Check sheet for the modelled part. Datum: model origin and axes. Units: mm. Face numbers are marked on the shaded views. A direction names the side the tool comes from. Coordinates: 2 decimals unless noted, no trailing zeros. Write each loop counter-clockwise with the first axis right and the second up, starting at its lowest first coordinate (ties: lowest second). Pieces come first, ordered by that corner, then holes. Notation, with made-up numbers: M 35.5,23 L 60.5,23 A31 cw 60.5,62 Z; hole C 71.25,33 d7. An arc over 180 degrees is marked long. Answer as CSV lines item,"result". Start each with the question number.
Q1. Thickness scan on line 1 along Z through (x, y) = (0, 6) (3 decimals); line 2 along Z through (x, y) = (0, 8.25) (3 decimals); line 3 along Y through (x, z) = (-2, 0) (1 decimal). Record the ranges inside material, lowest first. Write a range as from..to.
Q2. Sectioned sample at A-A, the plane y = 22.5. Record the cut outline in (x, z) (3 decimals).
Q3. Sectioned sample at D-D, the plane y = 63. Record the cut outline in (x, z) (1 decimal), then the cut area to 3 significant figures.
Q4. Depth check by flat-ended pin: pin 1 Ø18 at (y, z) = (65, 0.5) entering from -X; pin 2 Ø18 at (y, z) = (64, 5) entering from +X; pin 3 Ø8 at (x, z) = (-3.5, -4) entering from -Y. Enter the tip coordinate at first touch or a pass-through.
Q5. Mould release check, pull along Z, two halves, no side actions. Record for the marked faces 3, 4, 5 and 6: pulls with the +Z half, pulls with the -Z half, needs draft (parallel to the pull), parting line crosses it, or undercut.
Q6. Sectioned sample at C-C, the plane x = 0. Record the cut outline in (y, z) (1 decimal), then the cut area to 3 significant figures.
Q7. Access from +Z, -Z, +X, -X, +Y, -Y to the whole of each face (thin tool, end or side, straight path). Record for the marked faces 1 and 2.
Autodesk Fusion 360 part; units mm, degrees
sketch "Sketch1" plane through (0, 0, 0) normal (0, 1, 0) x (1, 0, 0)
  circle A0 centre (0, 0) radius 24.875
  line L0 (-23.4897, 87.6649) -> (23.4897, 87.6649)
  line L1 (23.4897, 87.6649) -> (64.1752, 64.1752)
  line L2 (64.1752, 64.1752) -> (87.6649, 23.4897)
  line L3 (87.6649, 23.4897) -> (87.6649, -23.4897)
  line L4 (87.6649, -23.4897) -> (64.1752, -64.1752)
  line L5 (64.1752, -64.1752) -> (23.4897, -87.6649)
  line L6 (23.4897, -87.6649) -> (-23.4897, -87.6649)
  line L7 (-23.4897, -87.6649) -> (-64.1752, -64.1752)
  line L8 (-64.1752, -64.1752) -> (-87.6649, -23.4897)
  line L9 (-87.6649, -23.4897) -> (-87.6649, 23.4897)
  line L10 (-87.6649, 23.4897) -> (-64.1752, 64.1752)
  line L11 (-64.1752, 64.1752) -> (-23.4897, 87.6649)
  line L12 (-87.6649, 0) -> (0, 0) construction
  line L13 (0, 0) -> (87.6649, 0) construction
  line L14 (0, 0) -> (0, -87.6649) construction
  line L15 (0, 0) -> (0, 87.6649) construction
  line L16 (-22.15, 82.6649) -> (22.15, 82.6649)
  line L17 (22.15, 82.6649) -> (60.5149, 60.5149)
  line L18 (60.5149, 60.5149) -> (82.6649, 22.15)
  line L19 (82.6649, 22.15) -> (82.6649, -22.15)
  line L20 (82.6649, -22.15) -> (60.5149, -60.5149)
  line L21 (60.5149, -60.5149) -> (22.15, -82.6649)
  line L22 (22.15, -82.6649) -> (-22.15, -82.6649)
  line L23 (-22.15, -82.6649) -> (-60.5149, -60.5149)
  line L24 (-60.5149, -60.5149) -> (-82.6649, -22.15)
  line L25 (-82.6649, -22.15) -> (-82.6649, 22.15)
  line L26 (-82.6649, 22.15) -> (-60.5149, 60.5149)
  line L27 (-60.5149, 60.5149) -> (-22.15, 82.6649)
  line L28 (0, 0) -> (-82.6649, 0) construction
  line L29 (0, 0) -> (0, 82.6649) construction
  line L30 (0, 0) -> (82.6649, 0) construction
  line L31 (0, 0) -> (0, -82.6649) construction
  point P0 (24.875, 0)
  dimension "d1" = 49.75
  dimension "d3" = 150
  dimension "d4" = 62.7899
  dimension "d5" = 5
  dimension "d9" = 150
  dimension "d10" = 44.3
extrude "Extrude1" add sketch "Sketch1" along normal blind 8 contours L16 L17 L18 L19 L20 L21 L22 L23 L24 L25 L26 L27
extrude "Extrude6" add sketch "Sketch1" along normal blind 28 contours L0 L1 L2 L3 L4 L5 L6 L7 L8 L9 L10 L11
extrude "Extrude2" add sketch "Sketch1" along normal blind 33 contours A0
sketch "Sketch2" plane through (0, 33, 0) normal (0, 1, 0) x (-1, 0, 0)
  circle A0 centre (0, 0) radius 24.875
  circle A1 centre (0, 0) radius 12.4375
  dimension "d15" = 49.75
  dimension "d16" = 24.875
extrude "Extrude3" add sketch "Sketch2" along normal blind 20 contours A1
sketch "Sketch3" plane through (0, 0, 0) normal (1, 0, 0) x (0, 0, -1)
  line L0 (12.4375, 53) -> (-12.4375, 53)
  line L1 (-12.4375, 33) -> (12.4375, 33)
  line L2 (0, 53) -> (0, 65.4375) construction
  circle A0 centre (0, 65.4375) radius 12.4375
  circle A1 centre (0, 65.4375) radius 8
  line L3 (0, 65.4375) -> (-12.4375, 65.4375) construction
  line L4 (0, 65.4375) -> (12.4375, 65.4375) construction
  line L5 (-12.4375, 65.4375) -> (-12.4375, 53)
  line L6 (12.4375, 65.4375) -> (12.4375, 53)
  dimension "d19" = 24.875
  dimension "d20" = 16
  dimension "d21" = 24.875
extrude "Extrude4" add sketch "Sketch3" along normal mid plane 10
extrude "Extrude5" cut 1 faces at (20.5903, 33, 1.8537) along direction (0, 1, 0) blind 50
fillet "Fillet1" radius 2 2 edges at (5, 53, 0) (-5, 53, 0)
sketch "Sketch4" plane through (0, 0, 0) normal (0, -1, 0) x (1, 0, 0)
  line L0 (-87.6649, -23.4897) -> (-64.1752, -64.1752)
  line L1 (-64.1752, -64.1752) -> (-23.4897, -87.6649)
  line L2 (-23.4897, -87.6649) -> (23.4897, -87.6649)
  line L3 (23.4897, -87.6649) -> (64.1752, -64.1752)
  line L4 (64.1752, -64.1752) -> (87.6649, -23.4897)
  line L5 (87.6649, -23.4897) -> (87.6649, 23.4897)
  line L6 (87.6649, 23.4897) -> (64.1752, 64.1752)
  line L7 (64.1752, 64.1752) -> (23.4897, 87.6649)
  line L8 (23.4897, 87.6649) -> (-23.4897, 87.6649)
  line L9 (-23.4897, 87.6649) -> (-64.1752, 64.1752)
  line L10 (-64.1752, 64.1752) -> (-87.6649, 23.4897)
  line L11 (-87.6649, 23.4897) -> (-87.6649, -23.4897)
  line L12 (0, 87.6649) -> (0, -87.6649) construction
  line L13 (87.6649, 0) -> (-87.6649, 0) construction
  circle A0 centre (0, 0) radius 13.725
  dimension "d30" = 27.45
extrude "Extrude7" cut sketch "Sketch4" against normal blind 11 contours A0
equation "d9 = d3"
equation "d13 = d11 + 25 mm"
equation "d16 = d15 / 2"
equation "d19 = d21"
equation "d28 = d11 + 20 mm"
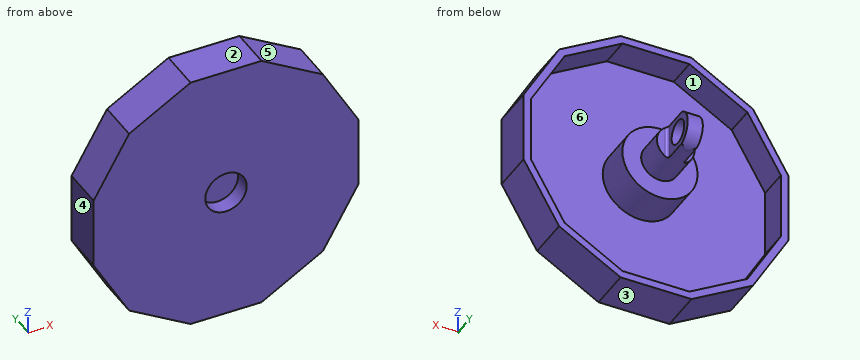
Output:
1,line 1,"z = -87.665..-13.725, 13.725..87.665"
1,line 2,"z = -87.665..-82.665, -24.875..-13.725, 13.725..24.875, 82.665..87.665"
1,line 3,"y = 11..57.4, 73.4..77.9"
2,outline,"M -87.665,-23.49 L -64.175,-64.175 L -23.49,-87.665 L 23.49,-87.665 L 64.175,-64.175 L 87.665,-23.49 L 87.665,23.49 L 64.175,64.175 L 23.49,87.665 L -23.49,87.665 L -64.175,64.175 L -87.665,23.49 Z; C 0,0 d49.75; hole M -82.665,-22.15 L -60.515,-60.515 L -22.15,-82.665 L 22.15,-82.665 L 60.515,-60.515 L 82.665,-22.15 L 82.665,22.15 L 60.515,60.515 L 22.15,82.665 L -22.15,82.665 L -60.515,60.515 L -82.665,22.15 Z"
3,outline,"M -5,-11.4 A12.4 ccw 5,-11.4 L 5,-7.6 L -5,-7.6 Z; M -5,7.6 L 5,7.6 L 5,11.4 A12.4 ccw -5,11.4 Z"
3,area,"89.5 mm^2"
4,pin 1,"stops at x = -5"
4,pin 2,"stops at x = 5"
4,pin 3,"stops at y = 11"
5,face 3,"pulls with the -Z half"
5,face 4,"needs draft"
5,face 5,"pulls with the +Z half"
5,face 6,"undercut"
6,outline,"M 0,-87.7 L 28,-87.7 L 28,-82.7 L 8,-82.7 L 8,-24.9 L 33,-24.9 L 33,-12.4 L 65.4,-12.4 A12.4 ccw 65.4,12.4 L 33,12.4 L 33,24.9 L 8,24.9 L 8,82.7 L 28,82.7 L 28,87.7 L 0,87.7 L 0,13.7 L 11,13.7 L 11,-13.7 L 0,-13.7 Z; hole C 65.4,0 d16"
6,area,"3,390 mm^2"
7,face 1,"+Y"
7,face 2,"+Z, +X, -X, +Y, -Y"
